Geometry check sheet. Reference: drawing and pictorial views, mm from the part's lowest x, y, z. Give positions to 0.01 mm unless a question says otherwise; leave off trailing zeros. Loops run counter-clockwise (first coordinate to the right, second up) from the corner with the lowest first, then second, coordinate; pieces in that order, holes last. Notation, with made-up numbers: (14, 67.25) -> (52, 67.25) arc R15 ccw to (52, 73.25) -> close; hole circle Ø5 at (-40, 8). An arc over 180 degrees is marked (long way). Answer in a Markdown table with one row per item. Add a question column.
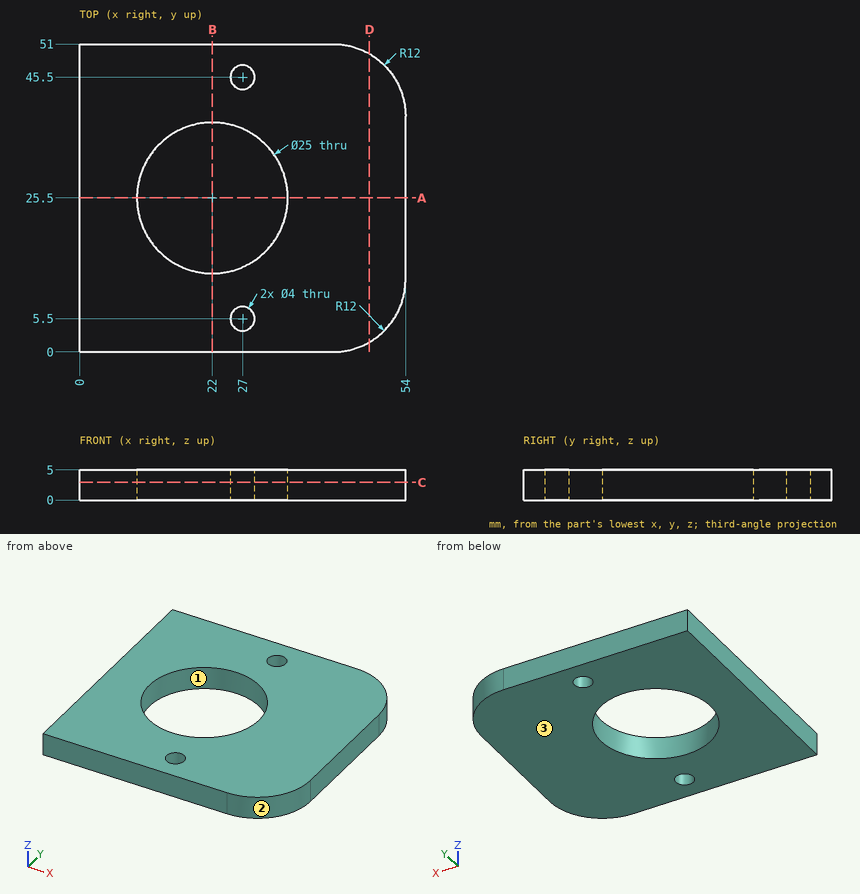
1. Sectioned sample at B-B (x = 22). Enter the section's corners in (y, z).
2. Material ranges on L1, parallel to Y at x = 22, z = 2.6; L2, parallel to Y at x = 27, z = 2.3; L3, parallel to Y at x = 15.5, z = 4.25, recorded low to high. Write a range as from..to.
3. Sectioned sample at A-A (y = 25.5). Enter the section's corners in (x, z), plus the area to 3 significant figures.
4. Release check for a two-part mould opening along Y. For the marked faces 1, 2 and 3 record: released by +Y, released by -Y, zero draft, split by the parting line, or undercut.
5. Gauge pin test, flat end, axial feed: pin 1 Ø1.5 at (x, z) = (44, 1.5) entering from -Y. Record the tip position at first contact, or that the pin passes through.
6. Sectioned sample at C-C (z = 2.95). Enter the section's corners in (x, y).
7. Sectioned sample at D-D (x = 48). Enter the section's corners in (y, z), plus the area to 3 significant figures.
Response:
| question | item | result |
|---|---|---|
| 1 | outline | (0, 0) -> (13, 0) -> (13, 5) -> (0, 5) -> close; (38, 0) -> (51, 0) -> (51, 5) -> (38, 5) -> close |
| 2 | L1 | y = 0..13, 38..51 |
| 2 | L2 | y = 0..3.5, 7.5..14.04, 36.96..43.5, 47.5..51 |
| 2 | L3 | y = 0..14.82, 36.18..51 |
| 3 | outline | (0, 0) -> (9.5, 0) -> (9.5, 5) -> (0, 5) -> close; (34.5, 0) -> (54, 0) -> (54, 5) -> (34.5, 5) -> close |
| 3 | area | 145 mm2 |
| 4 | face 1 | undercut |
| 4 | face 2 | released by -Y |
| 4 | face 3 | zero draft |
| 5 | pin 1 | stops at y = 0.07 |
| 6 | outline | (0, 0) -> (42, 0) arc R12 ccw to (54, 12) -> (54, 39) arc R12 ccw to (42, 51) -> (0, 51) -> close; hole circle Ø25 at (22, 25.5); hole circle Ø4 at (27, 5.5); hole circle Ø4 at (27, 45.5) |
| 7 | outline | (1.61, 0) -> (49.39, 0) -> (49.39, 5) -> (1.61, 5) -> close |
| 7 | area | 239 mm2 |
